Check sheet for the drawn part. Datum: minimum x, y, z corner. Units: mm. A direction names the side the tool comes from. Give positions to 0.01 mm unless a question says otherwise; leave off trailing zeros. Loops run counter-clockwise (first coordinate to the right, second up) from the corner with the lowest first, then second, coordinate; pieces in that order, holes last. Notation, with made-up numbers: (3, 48.5) - (62, 48.5) arc R16 ccw to (62, 79.5) - close; hole circle Ø2 at (82, 21). An arc over 180 degrees is marked (long way). Answer in a Markdown table with one row per item.
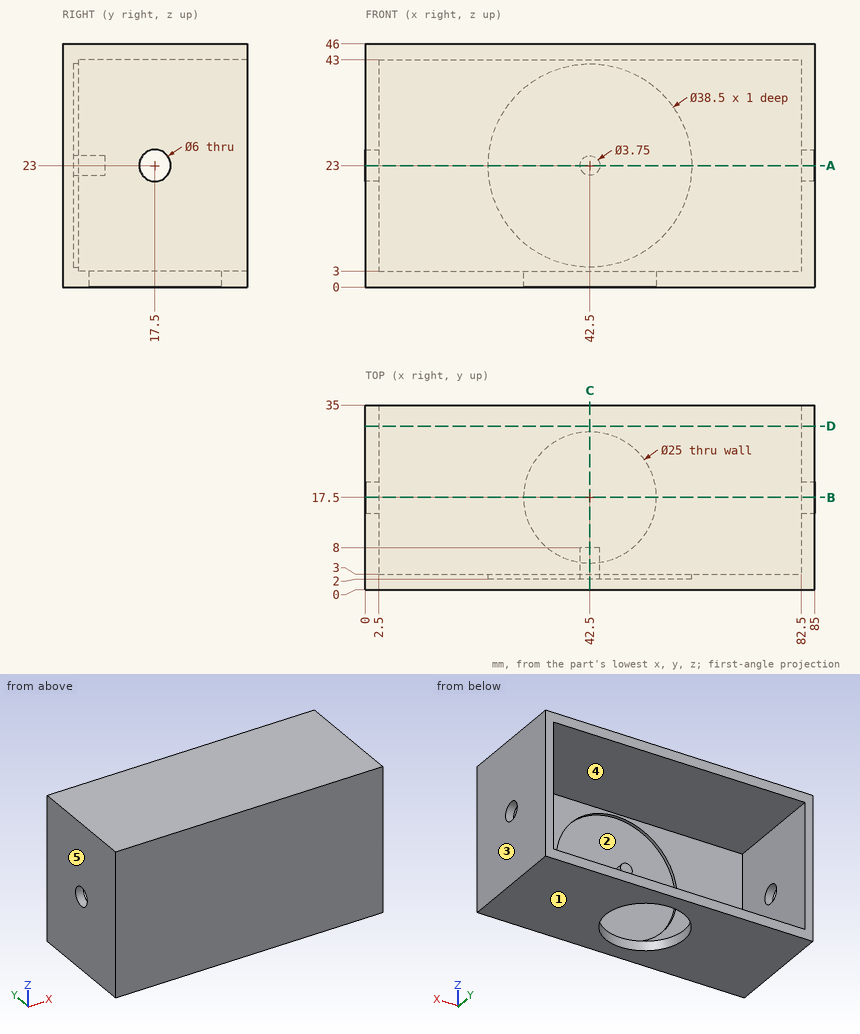
Q1. Sectioned sample at B-B (y = 17.5). Record the cut outline in (x, z), and give its area (3 significant figures).
Completed:
| item | result |
|---|---|
| outline | (0, 0) - (30, 0) - (30, 3) - (2.5, 3) - (2.5, 20) - (0, 20) - close; (0, 26) - (2.5, 26) - (2.5, 43) - (82.5, 43) - (82.5, 26) - (85, 26) - (85, 46) - (0, 46) - close; (55, 0) - (85, 0) - (85, 20) - (82.5, 20) - (82.5, 3) - (55, 3) - close |
| area | 605 mm^2 |
Q2. Thickness scan on line 1 (X direction, y = 2.7, z = 23) (3 decimals); line 2 (Z direction, x = 6, y = 7); line 3 (X direction, y = 17, z = 1). Record the ranges inside material, lowest first.
Completed:
| item | result |
|---|---|
| line 1 | 0 to 23.25, 40.625 to 44.375, 61.75 to 85 |
| line 2 | 0 to 3, 43 to 46 |
| line 3 | 0 to 30.01, 54.99 to 85 |
Q3. Sectioned sample at C-C (x = 42.5). Record the cut outline in (y, z) (3 decimals), and give its area (3 significant figures).
Completed:
| item | result |
|---|---|
| outline | (0, 0) - (5, 0) - (5, 3) - (3, 3) - (3, 3.75) - (2, 3.75) - (2, 21.125) - (8, 21.125) - (8, 24.875) - (2, 24.875) - (2, 42.25) - (3, 42.25) - (3, 43) - (35, 43) - (35, 46) - (0, 46) - close; (30, 0) - (35, 0) - (35, 3) - (30, 3) - close |
| area | 239 mm^2 |
Q4. Sectioned sample at A-A (z = 23). Record the cut outline in (x, y) (3 decimals).
Completed:
| item | result |
|---|---|
| outline | (0, 0) - (85, 0) - (85, 14.5) - (82.5, 14.5) - (82.5, 3) - (61.75, 3) - (61.75, 2) - (44.375, 2) - (44.375, 8) - (40.625, 8) - (40.625, 2) - (23.25, 2) - (23.25, 3) - (2.5, 3) - (2.5, 14.5) - (0, 14.5) - close; (0, 20.5) - (2.5, 20.5) - (2.5, 35) - (0, 35) - close; (82.5, 20.5) - (85, 20.5) - (85, 35) - (82.5, 35) - close |
Q5. Tool access check on the marked faces 4 and 5. Record the directions out of +Z, -Z, +X, -X, +Y, -Y that give a thin tool (end or side, any length) a straight path to the whole face; none if there is none.
Completed:
| item | result |
|---|---|
| face 4 | +Y |
| face 5 | +Z, -Z, -X, +Y, -Y |
Q6. Go/stop test with flat-tipped pins: P1, Ø1.1, axis at x = 42, z = 22.5, coming from the +Y side; P2, Ø1, axis at x = 25.5, z = 11.5, coming from the +Y side. Record where each tip stops, or that it passes through.
Completed:
| item | result |
|---|---|
| P1 | y = 8 |
| P2 | y = 3 |
Q7. Draft check along X on the marked faces 1, 2 and 3. Enter one of: +X half, -X half, draft (parallel to the pull), parting line (faces both ways), or undercut.
Completed:
| item | result |
|---|---|
| face 1 | draft |
| face 2 | undercut |
| face 3 | +X half |
Q8. Sectioned sample at D-D (y = 31). Record the cut outline in (x, z).
Completed:
| item | result |
|---|---|
| outline | (0, 0) - (85, 0) - (85, 46) - (0, 46) - close; hole (2.5, 3) - (82.5, 3) - (82.5, 43) - (2.5, 43) - close |
